Part model, mm, in its own coordinate system. Face numbers are marked on the shaded views. A direction names the side the tool comes from. Round coordinates to 2 decimals unless told otherwise and drop trailing zeros. Write each loop counter-clockwise with the first axis right and the second up, starting at its lowest first coordinate (ties: lowest second). Pieces come first, ordered by that corner, then holes. Notation, with made-up numbers: (24.25, -11) -> (53.25, -11) arc R23 cw to (53.25, 14) -> close; hole circle Ø3 at (11.5, 3.5). An arc over 180 degrees is marked (long way). Return JSON: item names as keys, results as strings. Group by question number.
```python
from build123d import *

# Parameters (mm, degrees)
SKETCH1_R                  = 13.8
BOSS_EXTRUDE1_DEPTH        = 37.8
SKETCH2_R                  = 4.965
BOSS_EXTRUDE2_DEPTH        = 2.58
SKETCH3_R                  = 4.3
CUT_EXTRUDE1_DEPTH         = 0.46
SKETCH4_R                  = 1.15
BOSS_EXTRUDE3_DEPTH        = 7.3
M2_5_CLEARANCE_HOLE1_D     = 2.9
M2_5_CLEARANCE_HOLE1_DEPTH = 10
M2_5_CLEARANCE_HOLE1_TIP   = 0.871247898
BOSS_EXTRUDE4_DEPTH        = 9


with BuildPart() as part:
    # Sketch1 → Boss-Extrude1 (new body)
    with BuildSketch(Plane(origin=(0, 0, 0), x_dir=(0, 0, -1), z_dir=(1, 0, 0))):
        Circle(SKETCH1_R)
    extrude(amount=BOSS_EXTRUDE1_DEPTH)

    # Sketch2 → Boss-Extrude2 (add)
    with BuildSketch(Plane(origin=(37.8, 0, 0), x_dir=(0, 0, -1), z_dir=(1, 0, 0))):
        Circle(SKETCH2_R)
    extrude(amount=BOSS_EXTRUDE2_DEPTH)

    # Sketch3 → Cut-Extrude1 (cut)
    with BuildSketch(Plane(origin=(40.38, 0, 0), x_dir=(0, 0, -1), z_dir=(1, 0, 0))):
        Circle(SKETCH3_R)
    extrude(amount=-CUT_EXTRUDE1_DEPTH, mode=Mode.SUBTRACT)

    # Sketch4 → Boss-Extrude3 (add)
    with BuildSketch(Plane(origin=(39.92, 0, 0), x_dir=(0, 0, -1), z_dir=(1, 0, 0))):
        Circle(SKETCH4_R)
    extrude(amount=BOSS_EXTRUDE3_DEPTH)

    # M2.5 Clearance Hole1
    with Locations(Plane(origin=(37.8, 0, 0), x_dir=(0, 0, -1), z_dir=(1, 0, 0))):
        with Locations((-8.05, 0), (8.05, 0)):
            Hole(M2_5_CLEARANCE_HOLE1_D / 2, depth=M2_5_CLEARANCE_HOLE1_DEPTH)
            with Locations((0, 0, -(M2_5_CLEARANCE_HOLE1_DEPTH + M2_5_CLEARANCE_HOLE1_TIP / 2))):  # 118° drill point
                Cone(0, M2_5_CLEARANCE_HOLE1_D / 2, M2_5_CLEARANCE_HOLE1_TIP, mode=Mode.SUBTRACT)

    # Sketch7 → Boss-Extrude4 (add)
    with BuildSketch(Plane.ZY):
        Polygon((-13.48707523, 2.922122814), (13.8, 0), (13.303912233, -3.666867776), (-12.668048772, -5.47362223), align=None)
    extrude(amount=BOSS_EXTRUDE4_DEPTH)


solid = part.part
```
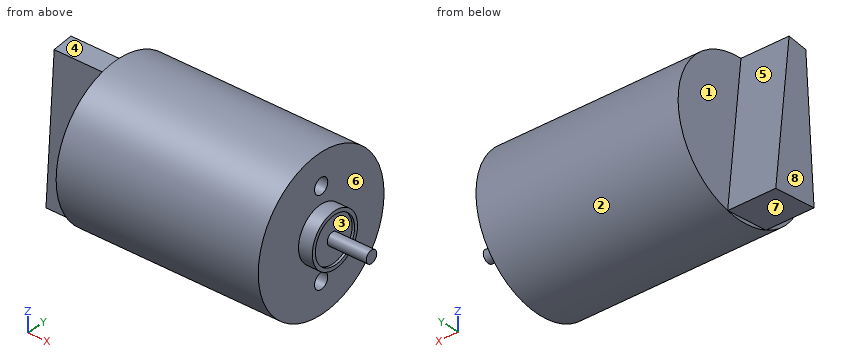
Item 1: Wall check: L1, parallel to Y at x = 40, z = 0 (3 decimals); L2, parallel to Z at x = 33.5, y = 0; L3, parallel to X at y = 5.25, z = 2.5. Give the ranges that are in metal, low to high.
Item 2: Flat gauge pins, fed straight in: P1, Ø2, axis at x = 34.5, y = -5.5, coming from the +Z side; P2, Ø1.5, axis at y = -6, z = 7, coming from the +X side; P3, Ø3, axis at x = 0.5, z = -10, coming from the -Y side. Where does each tip first touch, or does it go through?
Item 3: Cut at D-D (x = 20). Write the cut outline in (y, z).
Item 4: Cut at C-C (z = 0). Write the cut outline in (x, y) (3 decimals).
Item 5: Which spindle directions (+Z, -Z, +X, -X, +Y, -Y) get a long thin tool onto all of the face, cutting with end or side? Do the marked faces 4, 5, 6, 7 and 8. Say none if no direction does.
Item 6: Cut at B-B (y = 2.25). Write the cut outline in (x, z).
Item 7: Two-plate mould, pull along Z, no slides. Class the marked faces 1, 2 and 3: released by +Z, released by -Z, zero draft, split by the parting line, or undercut.
Item 8: Cut at A-A (x = 37). Write the cut outline in (y, z), then the cut area to 3 significant figures.
Checks:
{
 "1": {"L1": "y = -4.965 to -4.3, -1.15 to 1.15, 4.3 to 4.965", "L2": "z = -13.8 to -9.5, -6.6 to 6.6, 9.5 to 13.8", "L3": "x = 0 to 37.8"},
 "2": {"P1": "stops at z = 13.05", "P2": "stops at x = 37.8", "P3": "stops at y = -10.87"},
 "3": {"outline": "circle Ø27.6 at (0, 0)"},
 "4": {"outline": "(-9, -4.592) -> (0, -4.592) -> (0, -13.8) -> (37.8, -13.8) -> (37.8, -4.965) -> (40.38, -4.965) -> (40.38, -4.3) -> (39.92, -4.3) -> (39.92, -1.15) -> (47.22, -1.15) -> (47.22, 1.15) -> (39.92, 1.15) -> (39.92, 4.3) -> (40.38, 4.3) -> (40.38, 4.965) -> (37.8, 4.965) -> (37.8, 13.8) -> (0, 13.8) -> (0, 1.478) -> (-9, 1.478) -> close"},
 "5": {"face 4": "+Z, -X, -Y", "face 5": "+Z, -X, +Y", "face 6": "+X", "face 7": "-Z, -X, -Y", "face 8": "+Z, -Z, -X, +Y, -Y"},
 "6": {"outline": "(-9, -13.42) -> (0, -13.42) -> (0, -13.62) -> (37.8, -13.62) -> (37.8, -4.43) -> (40.38, -4.43) -> (40.38, -3.66) -> (39.92, -3.66) -> (39.92, 3.66) -> (40.38, 3.66) -> (40.38, 4.43) -> (37.8, 4.43) -> (37.8, 13.62) -> (0, 13.62) -> (0, -7.21) -> (-9, -7.21) -> close"},
 "7": {"face 1": "zero draft", "face 2": "split by the parting line", "face 3": "undercut"},
 "8": {"outline": "circle Ø27.6 at (0, 0); hole circle Ø2.9 at (0, -8.05); hole circle Ø2.9 at (0, 8.05)", "area": "585 mm2"}
}
